```python
from build123d import *

# Parameters (mm, degrees)
BOSS_EXTRUDE1_DEPTH     = 3.175
CUT_EXTRUDE1_DEPTH      = 272.1390812
CUT_EXTRUDE1_DEPTH_BACK = 272.1390812
CUT_EXTRUDE3_DEPTH      = 272.1390812
CUT_EXTRUDE3_DEPTH_BACK = 272.1390812


with BuildPart() as part:
    # Sketch1 → Boss-Extrude1 (new body)
    with BuildSketch(Plane(origin=(0, 0, 0), x_dir=(1, 0, 0), z_dir=(0, 1, 0))):
        Polygon((-244.348, 114.3), (244.348, 114.3), (244.348, 31.75), (244.348, -114.3), (241.173, -114.3), (209.931, -114.3), (209.931, -117.475), (178.181, -117.475), (178.181, -114.3), (112.903, -114.3), (112.903, -117.475), (81.153, -117.475), (81.153, -114.3), (15.875, -114.3), (15.875, -117.475), (-15.875, -117.475), (-15.875, -114.3), (-81.153, -114.3), (-81.153, -117.475), (-112.903, -117.475), (-112.903, -114.3), (-178.181, -114.3), (-178.181, -117.475), (-209.931, -117.475), (-209.931, -114.3), (-241.173, -114.3), (-244.348, -114.3), (-244.348, 31.75), align=None)
    extrude(amount=BOSS_EXTRUDE1_DEPTH)

    # Sketch2 → Cut-Extrude1 (cut, two sides: drawn at the far end of the back side and taken through both)
    with BuildSketch(Plane(origin=(0, 3.175, 0), x_dir=(1, 0, 0), z_dir=(0, 1, 0)).offset(-CUT_EXTRUDE1_DEPTH_BACK)):
        with BuildLine():
            Line((244.348, 27.94), (243.713, 27.94))
            ThreePointArc((243.713, 27.94), (241.916948776, 27.196051224), (241.173, 25.4))
            Line((241.173, 25.4), (241.173, -106.68))
            ThreePointArc((241.173, -106.68), (241.916948776, -108.476051224), (243.713, -109.22))
            Line((243.713, -109.22), (244.348, -109.22))
            Line((244.348, -109.22), (244.348, 27.94))
        make_face()
        with BuildLine():
            Line((-243.713, -109.22), (-244.348, -109.22))
            Line((-244.348, -109.22), (-244.348, 27.94))
            Line((-244.348, 27.94), (-243.713, 27.94))
            ThreePointArc((-243.713, 27.94), (-241.916948776, 27.196051224), (-241.173, 25.4))
            Line((-241.173, 25.4), (-241.173, -106.68))
            ThreePointArc((-241.173, -106.68), (-241.916948776, -108.476051224), (-243.713, -109.22))
        make_face()
    extrude(amount=CUT_EXTRUDE1_DEPTH + CUT_EXTRUDE1_DEPTH_BACK, mode=Mode.SUBTRACT)

    # Sketch4 → Cut-Extrude3 (cut, two sides: drawn at the far end of the back side and taken through both)
    with BuildSketch(Plane(origin=(0, 3.175, 0), x_dir=(1, 0, 0), z_dir=(0, 1, 0)).offset(-CUT_EXTRUDE3_DEPTH_BACK)):
        Polygon((-145.542, 27.94), (-147.1295, 27.94), (-147.1295, -109.22), (-145.542, -109.22), (-143.9545, -109.22), (-143.9545, 27.94), align=None)
        Polygon((-50.1015, -109.22), (-48.514, -109.22), (-46.9265, -109.22), (-46.9265, 27.94), (-48.514, 27.94), (-50.1015, 27.94), align=None)
        Polygon((46.9265, -109.22), (48.514, -109.22), (50.1015, -109.22), (50.1015, 27.94), (48.514, 27.94), (46.9265, 27.94), align=None)
        Polygon((143.9545, -109.22), (145.542, -109.22), (147.1295, -109.22), (147.1295, 27.94), (145.542, 27.94), (143.9545, 27.94), align=None)
    extrude(amount=CUT_EXTRUDE3_DEPTH + CUT_EXTRUDE3_DEPTH_BACK, mode=Mode.SUBTRACT)


solid = part.part
```
Read the model definition and answer for the solid it produces. Units are mm, in the model's axes. Coordinates: 2 decimals unless noted, no trailing zeros. Write each loop counter-clockwise with the first axis right and the second up, starting at its lowest first coordinate (ties: lowest second). Pieces come first, ordered by that corner, then holes. Notation, with made-up numbers: (42, 79.5) -> (74, 79.5) arc R34 ccw to (74, 116.5) -> close; hole circle Ø2 at (75, -26.75). An arc over 180 degrees is marked (long way). Write item = value, one per line.
(1) Straight lines are drawn through the part: L1, parallel to X at y = 1.3, z = -5; L2, parallel to Z at x = -80, y = 1.8. For each, find the intervals that lie inside material, in ascending order. Write a range as from..to.
From the geometry:
L1 = -241.17..-147.13, -143.95..-50.1, -46.93..46.93, 50.1..143.95, 147.13..241.17
L2 = -114.3..114.3
(2) Given pin 1 Ø1.6 at (y, z) = (2, 59.5) entering from +X; pin 2 Ø1.6 at (y, z) = (2.5, 116.5) entering from -X; pin 3 Ø1 at (x, y) = (154, 2) entering from +Z, each flat-ended and moving along its own axis, determine where each tip first touches the part or whether it passes through.
From the geometry:
pin_1 = 241.17
pin_2 = -209.93
pin_3 = 114.3
(3) Section A-A on z = 1 is taken. Write down the section's boundary in (x, y) (1 decimal), plus the area to 3 significant figures.
From the geometry:
outline = (-241.2, 0) -> (-147.1, 0) -> (-147.1, 3.2) -> (-241.2, 3.2) -> close; (-144, 0) -> (-50.1, 0) -> (-50.1, 3.2) -> (-144, 3.2) -> close; (-46.9, 0) -> (46.9, 0) -> (46.9, 3.2) -> (-46.9, 3.2) -> close; (50.1, 0) -> (144, 0) -> (144, 3.2) -> (50.1, 3.2) -> close; (147.1, 0) -> (241.2, 0) -> (241.2, 3.2) -> (147.1, 3.2) -> close
area = 1,490 mm2
(4) Section B-B on y = 1.7 is taken. Count the separate pieces of the cut face and the enclosed holes in it, plus the area to 3 significant figures.
From the geometry:
separate_pieces = 1
enclosed_holes = 4
area = 110,000 mm2
